Verification items for this drawing (mm, ordinates from the low corner). A direction names the side the tool comes from. Round coordinates to 2 decimals unless told otherwise and drop trailing zeros. Order: outer loops, then holes, each group sorted by start corner. A loop starts at its lowest first (then second) coordinate and runs counter-clockwise, first axis right, second up. Notation, with made-up numbers: M -38,86 L -32,86 A22 cw -32,125 Z; hole C 78,7 d2. An arc over 180 degrees is marked long. One line per item, written item: value. Start each with the question number.
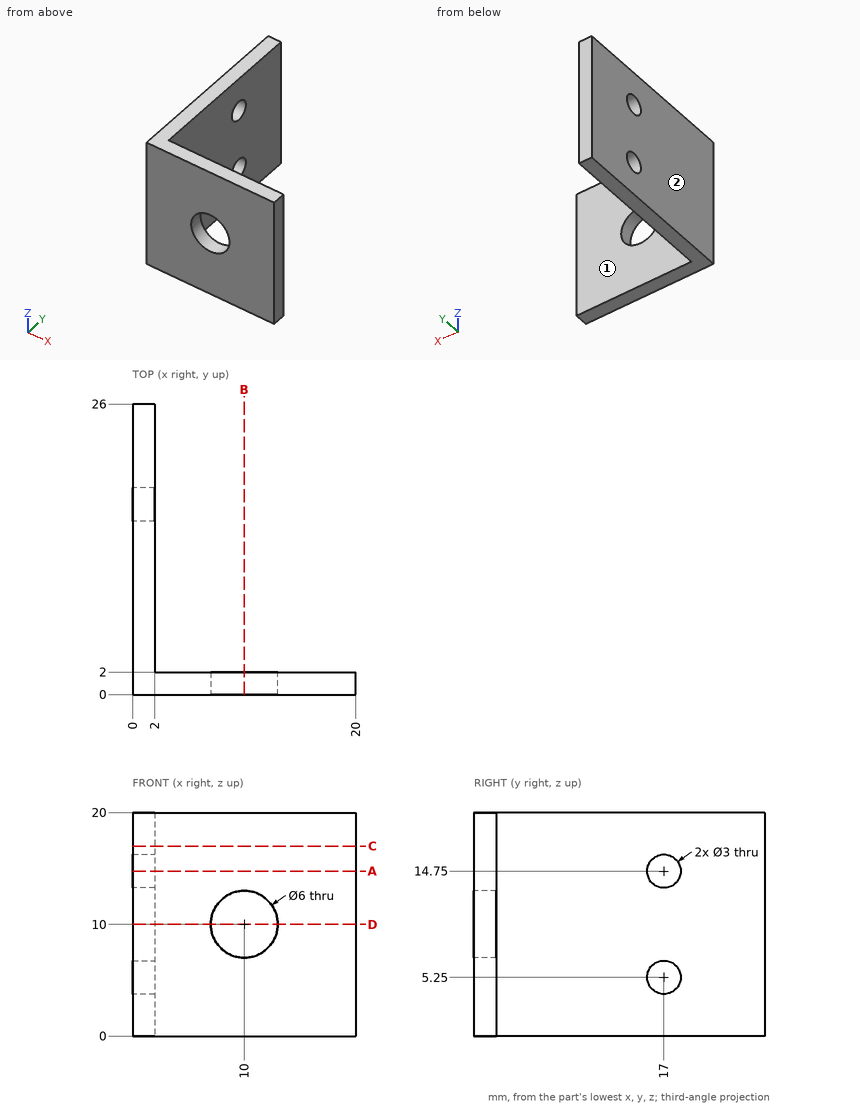
1. Section check C-C (z = 17). Record the cut outline in (x, y), and give its area (3 significant figures).
2. Scan lines: line 1 along Z through (x, y) = (10, 0.65); line 2 along Y through (x, z) = (1.65, 14.75); line 3 along X through (y, z) = (3.25, 8.5). Record each from-to range of solid material in increasing order.
3. Section check A-A (z = 14.75). Record the cut outline in (x, y).
4. Section check B-B (x = 10). Record the cut outline in (y, z), and give its area (3 significant figures).
5. Tool access check on the marked faces 1 and 2. Record the directions out of +Z, -Z, +X, -X, +Y, -Y that give a thin tool (end or side, any length) a straight path to the whole face; none if there is none.
6. Section check D-D (z = 10). Record the cut outline in (x, y).
7. Depth check by flat-ended pin: pin 1 (4 mm diameter, centred on y = 18.5, z = 16, fed in from -X); pin 2 (10 mm diameter, centred on y = 8, z = 13, fed in from +X); pin 3 (1.5 mm diameter, centred on x = 11.5, z = 12, fed in from +Y). Enter the tip coordinate at first touch or a pass-through.
Geometry check:
1. outline: M 0,0 L 20,0 L 20,2 L 2,2 L 2,26 L 0,26 Z
1. area: 88.0 mm²
2. line 1: z = 0 to 7, 13 to 20
2. line 2: y = 0 to 15.5, 18.5 to 26
2. line 3: x = 0 to 2
3. outline: M 0,0 L 20,0 L 20,2 L 2,2 L 2,15.5 L 0,15.5 Z; M 0,18.5 L 2,18.5 L 2,26 L 0,26 Z
4. outline: M 0,0 L 2,0 L 2,7 L 0,7 Z; M 0,13 L 2,13 L 2,20 L 0,20 Z
4. area: 28.0 mm²
5. face 1: +Z, -Z, +X, +Y
5. face 2: +Z, -Z, -X, +Y, -Y
6. outline: M 0,0 L 7,0 L 7,2 L 2,2 L 2,26 L 0,26 Z; M 13,0 L 20,0 L 20,2 L 13,2 Z
7. pin 1: stops at x = 0
7. pin 2: stops at x = 2
7. pin 3: stops at y = 2
